Work out the finished part from the listing and answer in its coordinate system (mm). A direction names the side the tool comes from. Round coordinates to 2 decimals unless told otherwise and drop trailing zeros. Loops run counter-clockwise (first coordinate to the right, second up) from the corner with the lowest first, then second, coordinate; pieces in that order, holes last.
```python
from build123d import *

# Parameters (mm, degrees)
ESQUISSE1_R    = 1
CORPS_DEPTH    = 8
ESQUISSE2_R    = 2
APPUIS_DEPTH   = 0.14
TETE_DEPTH     = 1.26
CHANFREIN_SIZE = 0.25


with BuildPart() as part:
    # Esquisse1 → CORPS (new body)
    with BuildSketch(Plane(origin=(0, 0, 0), x_dir=(1, 0, 0), z_dir=(0, 1, 0))):
        with Locations(Location((0, 0, 0), (0, 0, 270))):
            Circle(ESQUISSE1_R)
    extrude(amount=CORPS_DEPTH)

    # Esquisse2 → APPUIS (add)
    with BuildSketch(Plane(origin=(0, 0, 0), x_dir=(-1, 0, 0), z_dir=(0, -1, 0))):
        with Locations(Location((0, 0, 0), (0, 0, 90))):
            Circle(ESQUISSE2_R)
    extrude(amount=APPUIS_DEPTH)

    # Esquisse3 → TETE (add)
    with BuildSketch(Plane(origin=(0, -0.14, 0), x_dir=(-1, 0, 0), z_dir=(0, -1, 0))):
        Polygon((0, -2.309401077), (2, -1.154700538), (2, 1.154700538), (0, 2.309401077), (-2, 1.154700538), (-2, -1.154700538), align=None)
    extrude(amount=TETE_DEPTH)

    # Esquisse4 → CHANFREIN_TETE (revolve, cut)
    with BuildSketch(Plane(origin=(0, 0, 0), x_dir=(0, 0, -1), z_dir=(1, 0, 0)), mode=Mode.PRIVATE) as chanfrein_tete_sk:
        Polygon((2.309401077, -1.2), (2.109401077, -1.4), (2.309401077, -1.4), align=None)
    revolve(chanfrein_tete_sk.sketch.rotate(Axis((0, 0, 0), (0, -1, 0)), 210), axis=Axis((0, 0, 0), (0, -1, 0)), mode=Mode.SUBTRACT)

    # CHANFREIN
    chanfrein_edges = [part.edges().sort_by_distance(p)[0] for p in [
        (0, 8, -1),
    ]]
    chamfer(chanfrein_edges, length=CHANFREIN_SIZE)


solid = part.part
```
1. Given pin 1 (0.8 mm diameter, centred on x = 1.5, z = 0.5, fed in from +Y); pin 2 (1 mm diameter, centred on y = 5, z = 0, fed in from +X), each flat-ended and moving along its own axis, determine where each tip first touches the part or whether it passes through.
Answer key:
pin 1: stops at y = 0
pin 2: stops at x = 1
2. Consider probe 1 along Y at (x, z) = (-0.5, 1.65); probe 2 along Z at (x, y) = (-0.05, 1). Determine where each line is inside the solid, lowest interval first.
Answer key:
probe 1: y = -1.4 to 0
probe 2: z = -1 to 1
3. Which of the six approach directions +Z, -Z, +X, -X, +Y, -Y give full straight-line access (tool end or side, diameter ignored) to faces 1 (the face through (-1, 0, -1)), 2 (the face through (-2, -1, 0))?
Answer key:
face 1: +Y
face 2: +Z, -Z, -X, +Y, -Y
4. Find section B-B (y = 4.25). Write down the section's boundary in (x, z), then the cut area to 3 significant figures.
Answer key:
outline: circle Ø2 at (0, 0)
area: 3.14 mm2
